```python
from build123d import *

# Parameters (mm, degrees)
SKETCH1_R               = 88.9
SKETCH1_R_2             = 85.725
BOSS_EXTRUDE1_DEPTH     = 301.625
CUT_EXTRUDE1_REACH      = 328.778
CUT_EXTRUDE1_END_RADIUS = 88.9
SKETCH2_W               = 127
SKETCH2_H               = 206.502
SKETCH2_H_2             = 320.548
CIRPATTERN1_COUNT       = 3


with BuildPart() as part:
    # Sketch1 → Boss-Extrude1 (new, symmetric)
    with BuildSketch(Plane(origin=(0, 0, 0), x_dir=(1, 0, 0), z_dir=(0, 1, 0))):
        with Locations(Location((0, 0, 0), (0, 0, 270))):
            Circle(SKETCH1_R)
        with Locations(Location((0, 0, 0), (0, 0, 270))):
            Circle(SKETCH1_R_2, mode=Mode.SUBTRACT)
    extrude(amount=BOSS_EXTRUDE1_DEPTH, both=True)

    # Cut-Extrude1: up to this cylinder (the profile starts inside it)
    cut_extrude1_end = Plane(origin=(0, -28.5115, 0), z_dir=(0, -1, 0)) * Cylinder(CUT_EXTRUDE1_END_RADIUS, 1125.281, mode=Mode.PRIVATE)
    # Sketch2 → Cut-Extrude1 (cut, up to the surface)
    with BuildSketch(Plane.XY, mode=Mode.PRIVATE) as cut_extrude1_sk1:
        with Locations((0, -172.974)):
            Rectangle(SKETCH2_W, SKETCH2_H)
    cut_extrude1_tool1 = extrude(cut_extrude1_sk1.sketch, amount=-CUT_EXTRUDE1_REACH, mode=Mode.PRIVATE) & cut_extrude1_end
    # Sketch2 → Cut-Extrude1 (cut, up to the surface)
    with BuildSketch(Plane.XY, mode=Mode.PRIVATE) as cut_extrude1_sk2:
        with Locations((0, 115.951)):
            Rectangle(SKETCH2_W, SKETCH2_H_2)
    cut_extrude1_tool2 = extrude(cut_extrude1_sk2.sketch, amount=-CUT_EXTRUDE1_REACH, mode=Mode.PRIVATE) & cut_extrude1_end
    cut_extrude1 = cut_extrude1_tool1.solids().sort_by_distance((0, -172.974, 0))[0] + cut_extrude1_tool2.solids().sort_by_distance((0, 115.951, 0))[0]
    add(cut_extrude1, mode=Mode.SUBTRACT)

    # CirPattern1: Cut-Extrude1 ×3 about axis
    cirpattern1_axis = Axis((0, 0, 0), (0, 1, 0))
    for i in range(1, CIRPATTERN1_COUNT):
        add(cut_extrude1.rotate(cirpattern1_axis, i * 360 / CIRPATTERN1_COUNT), mode=Mode.SUBTRACT)


solid = part.part
```
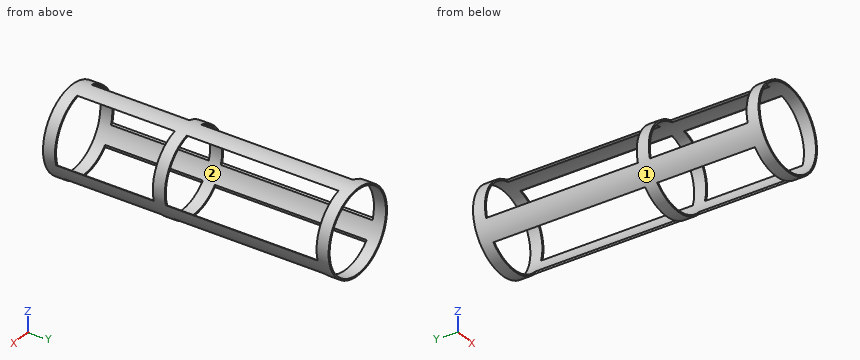
The model under review builds one solid part; all positions refer to its coordinate system, in mm. Face numbers are marked on the shaded views. Give positions to 0.01 mm unless a question says otherwise; leave off trailing zeros. Loops run counter-clockwise (first coordinate to the right, second up) from the corner with the lowest first, then second, coordinate; pieces in that order, holes last. Notation, with made-up numbers: (31.25, -21) - (75.25, -21) arc R19 cw to (75.25, 11) - close; hole circle Ø8 at (43, -38.5). An arc over 180 degrees is marked (long way). Answer as a JSON object with one key per item and string values.
Q1. Add section A-A on z = 0. State the section outline as (x, y) points (3 decimals), plus the area to 3 significant figures.
Worked out:
{"outline": "(-88.9, -301.625) - (-85.725, -301.625) - (-85.725, -276.225) - (-88.9, -276.225) - close; (-88.9, -69.723) - (-85.725, -69.723) - (-85.725, -44.323) - (-88.9, -44.323) - close; (-88.9, 276.225) - (-85.725, 276.225) - (-85.725, 301.625) - (-88.9, 301.625) - close; (85.725, -301.625) - (88.9, -301.625) - (88.9, -276.225) - (85.725, -276.225) - close; (85.725, -69.723) - (88.9, -69.723) - (88.9, -44.323) - (85.725, -44.323) - close; (85.725, 276.225) - (88.9, 276.225) - (88.9, 301.625) - (85.725, 301.625) - close", "area": "484 mm^2"}
Q2. Add section C-C on y = -3.5. State the section outline as (x, z) points (3 decimals).
Worked out:
{"outline": "(-85.632, -23.884) arc R88.9 ccw to (-63.5, -62.217) - (-63.5, -57.589) arc R85.725 cw to (-81.624, -26.198) - close; (-22.132, 86.101) - (-18.124, 83.787) arc R85.725 cw to (18.124, 83.787) - (22.132, 86.101) arc R88.9 ccw to start; (63.5, -62.217) arc R88.9 ccw to (85.632, -23.884) - (81.624, -26.198) arc R85.725 cw to (63.5, -57.589) - close"}
Q3. Mouldability with a two-part tool opening along X and no side actions: class the marked faces 1 and 2 as +X half, -X half, draft (parallel to the pull), parting line (faces both ways), or undercut.
Worked out:
{"face 1": "parting line", "face 2": "undercut"}
Q4. Add section D-D on z = -37.5. State the section outline as (x, y) points (3 decimals), plus the area to 3 significant figures.
Worked out:
{"outline": "(-80.604, -301.625) - (-77.088, -301.625) - (-77.088, 301.625) - (-80.604, 301.625) - close; (77.088, -301.625) - (80.604, -301.625) - (80.604, 301.625) - (77.088, 301.625) - close", "area": "4,240 mm^2"}
Q5. Add section B-B on x = -69. State the section outline as (y, z) points (3 decimals), plus the area to 3 significant figures.
Worked out:
{"outline": "(-301.625, -56.055) - (301.625, -56.055) - (301.625, -50.87) - (-301.625, -50.87) - close; (-301.625, 50.87) - (-276.225, 50.87) - (-276.225, 56.055) - (-301.625, 56.055) - close; (-69.723, 50.87) - (-44.323, 50.87) - (-44.323, 56.055) - (-69.723, 56.055) - close; (276.225, 50.87) - (301.625, 50.87) - (301.625, 56.055) - (276.225, 56.055) - close", "area": "3,520 mm^2"}
Q6. To check wall thickness, follow line 1 along X through (y, z) = (-52.5, 0) (3 decimals); line 2 along X through (y, z) = (277.5, -15); line 3 along Z through (x, y) = (0, 164.5) (3 decimals). State the ranges of each line that lie inside material, in increasing order.
Worked out:
{"line 1": "x = -88.9 to -85.725, 85.725 to 88.9", "line 2": "x = -87.63 to -84.4, 84.4 to 87.63", "line 3": "z = 85.725 to 88.9"}
Q7. Insertion check: pin 1 (8 mm diameter, centred on y = -68, z = 0, fed in from +X); pin 2 (21 mm diameter, centred on x = 59.5, z = 41, fed in from +Y); pin 3 (3.5 mm diameter, centred on y = 116, z = -59, fed in from +X); pin 4 (6 mm diameter, centred on y = -50, z = 2.5, fed in from -X). Each pin has a flat end and moves straight along its axis. Give the tip position at first contact, or say it passes through.
Worked out:
{"pin 1": "stops at x = 88.9", "pin 2": "passes through", "pin 3": "stops at x = 68.01", "pin 4": "stops at x = -88.9"}
